Job drawing, mm, ordinate dimensions from the low corner. One solid piece. A direction names the side the tool comes from. Give positions to 0.01 mm unless a question says otherwise; leave off trailing zeros. Order: outer loops, then holes, each group sorted by start corner. A loop starts at its lowest first (then second) coordinate and runs counter-clockwise, first axis right, second up.
Item 1: Band-saw the part on C-C on x = 6.25. Count the separate pieces of the cut face and the enclosed holes in it, plus the area to 3 significant figures.
Item 2: Wall check: L1, parallel to X at y = 1.9, z = 14.75; L2, parallel to Y at x = 4, z = 22; L3, parallel to X at y = 3.55, z = 7.95. Give the ranges that are in metal, low to high.
Item 3: Two-plate mould, pull along Z, no slides. Class the marked faces 3, 4 and 5: released by +Z, released by -Z, zero draft, split by the parting line, or undercut.
Item 4: Band-saw the part on B-B on z = 21.95. Give the cut face in (x, y).
Item 5: Band-saw the part on A-A on z = 14.75. Give the cut face in (x, y).
Item 6: Which spindle directions (+Z, -Z, +X, -X, +Y, -Y) get a long thin tool onto all of the face, cutting with end or side? Do the marked faces 1 and 2. Say none if no direction does.
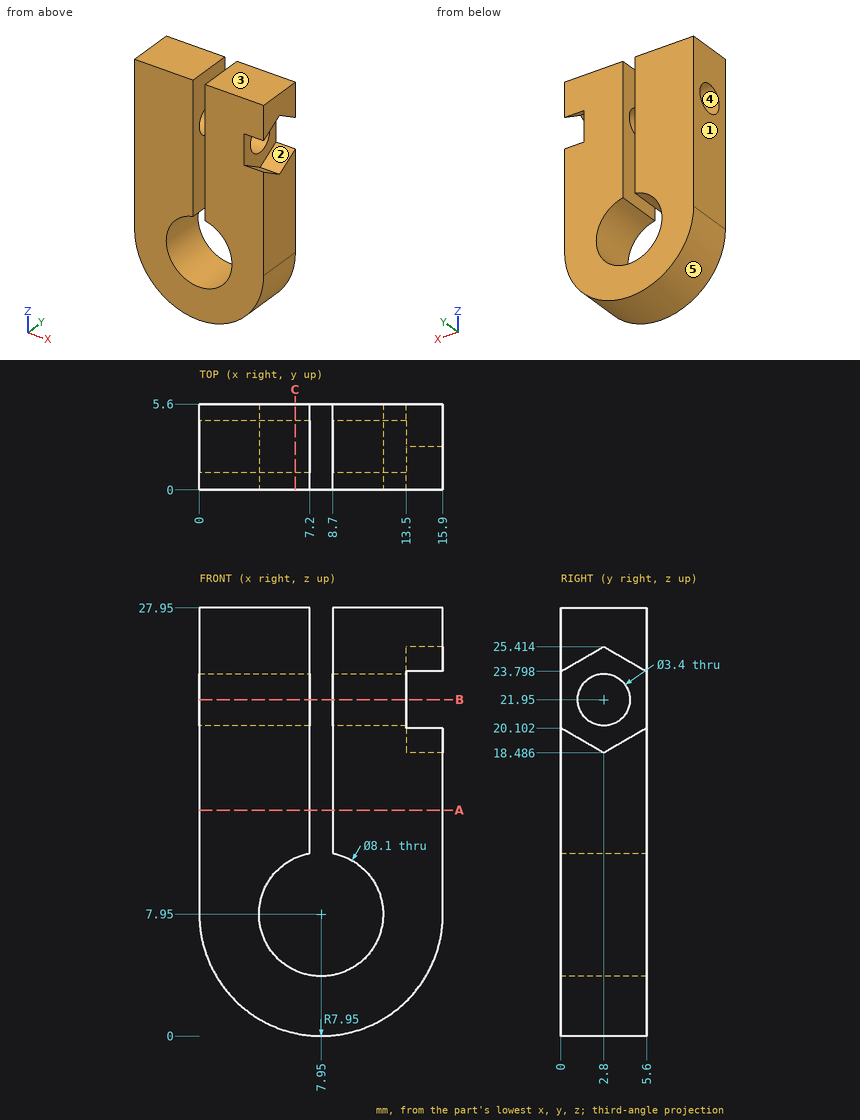
The answers:
1. separate pieces: 2
1. enclosed holes: 1
1. area: 105 mm2
2. L1: x = 0 to 7.2, 8.7 to 15.9
2. L2: y = 0 to 1.1, 4.5 to 5.6
2. L3: x = 0 to 3.9, 12 to 15.9
3. face 3: released by +Z
3. face 4: undercut
3. face 5: released by -Z
4. outline: (0, 0) - (7.2, 0) - (7.2, 1.1) - (0, 1.1) - close; (0, 4.5) - (7.2, 4.5) - (7.2, 5.6) - (0, 5.6) - close; (8.7, 0) - (13.5, 0) - (13.5, 1.1) - (8.7, 1.1) - close; (8.7, 4.5) - (13.5, 4.5) - (13.5, 5.6) - (8.7, 5.6) - close
5. outline: (0, 0) - (7.2, 0) - (7.2, 5.6) - (0, 5.6) - close; (8.7, 0) - (15.9, 0) - (15.9, 5.6) - (8.7, 5.6) - close
6. face 1: +Z, -Z, -X, +Y, -Y
6. face 2: +X
